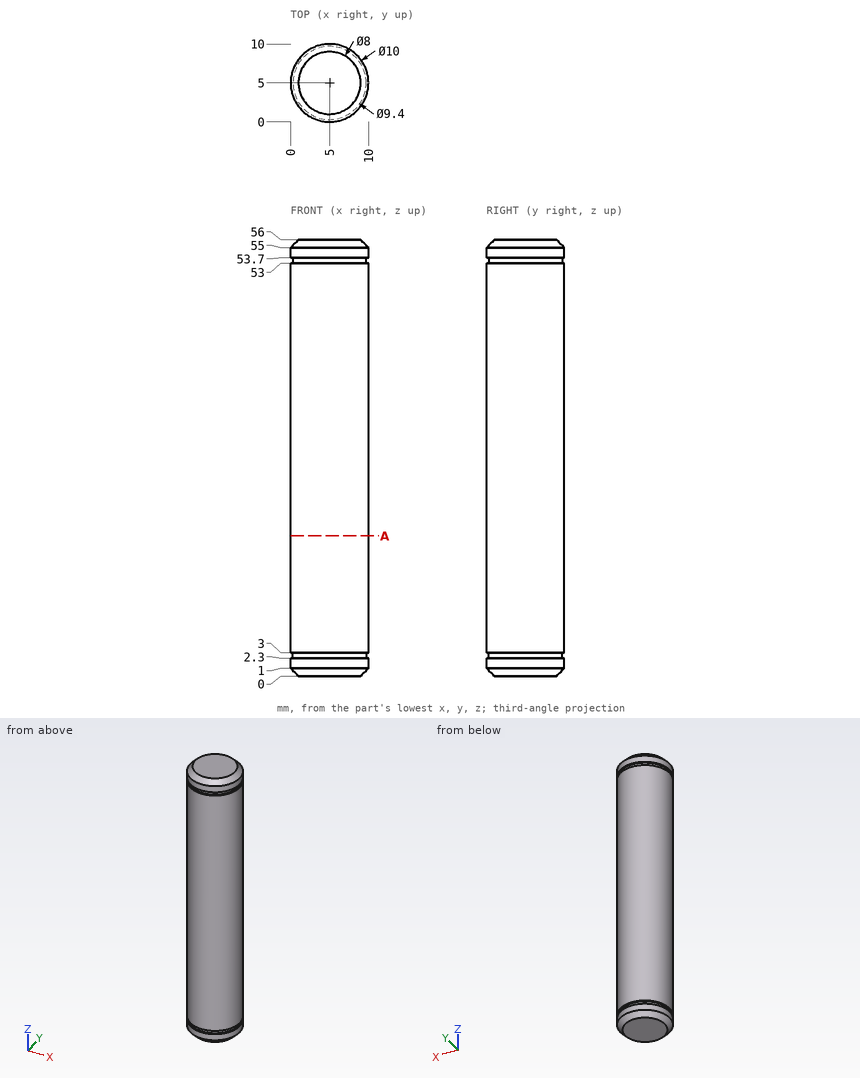
Part print with two shaded views. Sizes in mm from the minimum x, y, z corner. Round coordinates to 2 decimals unless told otherwise and drop trailing zeros. Loops run counter-clockwise (first coordinate to the right, second up) from the corner with the lowest first, then second, coordinate; pieces in that order, holes last.
1. Slice it at A-A (z = 18). Give the cut face in (x, y), and give its area (3 significant figures).
Solutions:
outline: circle Ø10 at (5, 5)
area: 78.5 mm2
2. Drill centre lines: line 1 along Z through (x, y) = (0.5, 6.75); line 2 along Y through (x, z) = (4.75, 3.5); line 3 along Y through (x, z) = (8, 7.5). Where is each one in solid material? Low to high.
Solutions:
line 1: z = 0.83 to 2.3, 3 to 53, 53.7 to 55.17
line 2: y = 0.01 to 9.99
line 3: y = 1 to 9
3. Flat gauge pins, fed straight in: pin 1 (2 mm diameter, centred on x = 7, y = 8.5, fed in from -Z); pin 2 (1 mm diameter, centred on x = 2.5, z = 43.5, fed in from -Y); pin 3 (5 mm diameter, centred on y = 2, z = 7, fed in from +X). Where does each tip first touch, or does it go through?
Solutions:
pin 1: stops at z = 0
pin 2: stops at y = 0.42
pin 3: stops at x = 9.97
